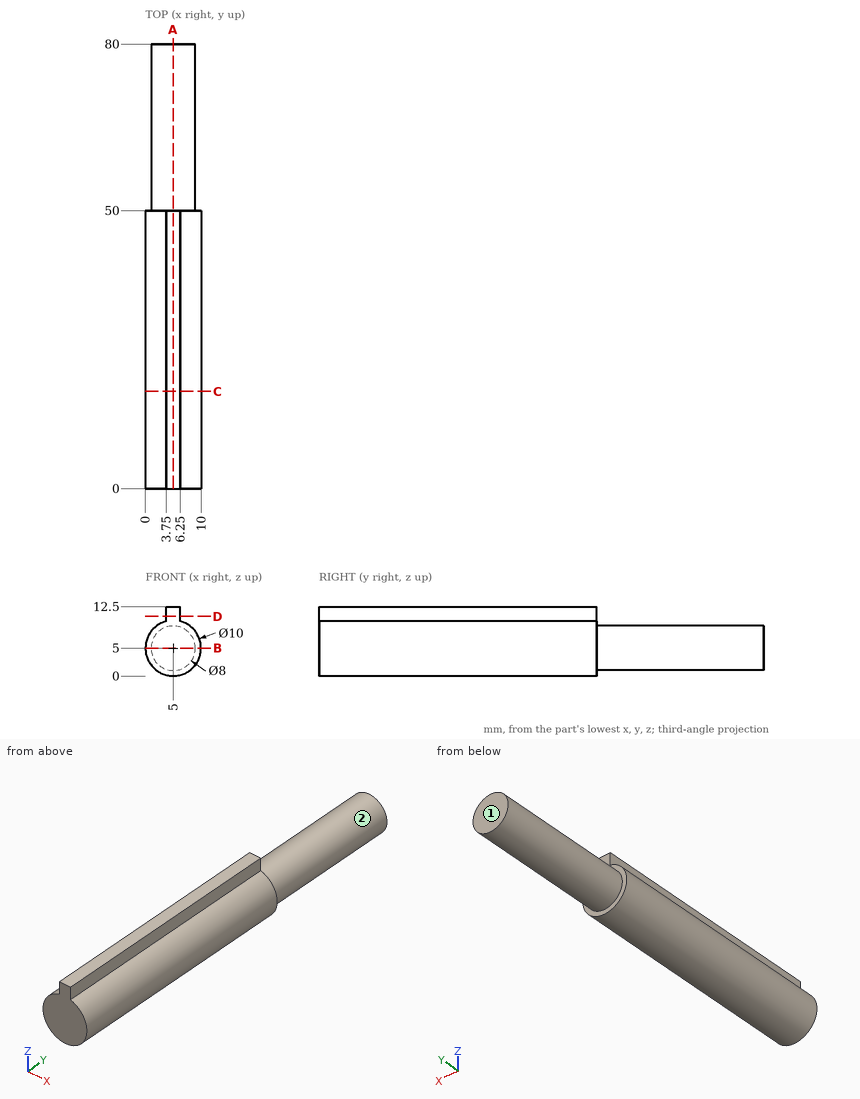
Geometry: see drawing. Coordinates: mm, zero at the bounding-box minimum. A direction names the side the tool comes from. Coordinates: 2 decimals unless noted, no trailing zeros. Loops run counter-clockwise (first coordinate to the right, second up) from the corner with the lowest first, then second, coordinate; pieces in that order, holes last. Notation, with made-up numbers: (1, 63) -> (55, 63) arc R4 ccw to (55, 68) -> close; hole circle Ø8 at (35, 29.25). An arc over 180 degrees is marked (long way). Use a Markdown table: item, result.
1) Cut plane B-B (z = 5). Return the cut outline in (x, y).
Results found:
| item | result |
|---|---|
| outline | (0, 0) -> (10, 0) -> (10, 50) -> (9, 50) -> (9, 80) -> (1, 80) -> (1, 50) -> (0, 50) -> close |
2) Contact query for flat-ended pins moving along their axis: pin 1 (5 mm diameter, centred on y = 56, z = 7.5, fed in from -X); pin 2 (2 mm diameter, centred on x = 5, y = 66.5, fed in from -Z); pin 3 (3 mm diameter, centred on y = 18.5, z = 12, fed in from -X). Output: stop coordinate, or through.
Results found:
| item | result |
|---|---|
| pin 1 | stops at x = 1 |
| pin 2 | stops at z = 1 |
| pin 3 | stops at x = 3.75 |
3) Cut plane C-C (y = 17.5). Return the cut outline in (x, z).
Results found:
| item | result |
|---|---|
| outline | (3.75, 9.84) arc R5 ccw (long way) to (6.25, 9.84) -> (6.25, 12.5) -> (3.75, 12.5) -> close |
4) Access query for the marked faces 1 and 2. Directions: +Z, -Z, +X, -X, +Y, -Y. A direction counts if a zero-diameter tool reaches every point of the face in a straight line with its end or side. Return the directions, or none.
Results found:
| item | result |
|---|---|
| face 1 | +Z, -Z, +X, -X, +Y |
| face 2 | +Y |
5) Cut plane D-D (z = 10.75). Return the cut outline in (x, y).
Results found:
| item | result |
|---|---|
| outline | (3.75, 0) -> (6.25, 0) -> (6.25, 50) -> (3.75, 50) -> close |
6) Material intervals for line 1 along Y through (x, z) = (1, 5.75); line 2 along X through (y, z) = (47, 10.5); line 3 along X through (y, z) = (27, 2), sorted ascending. Write a range as from..to.
Results found:
| item | result |
|---|---|
| line 1 | y = 0..50 |
| line 2 | x = 3.75..6.25 |
| line 3 | x = 1..9 |
7) Cut plane A-A (x = 5). Return the cut outline in (y, z).
Results found:
| item | result |
|---|---|
| outline | (0, 0) -> (50, 0) -> (50, 1) -> (80, 1) -> (80, 9) -> (50, 9) -> (50, 12.5) -> (0, 12.5) -> close |
